Check sheet for the drawn part. Datum: minimum x, y, z corner. Units: mm. A direction names the side the tool comes from. Coordinates: 2 decimals unless noted, no trailing zeros. Loops run counter-clockwise (first coordinate to the right, second up) from the corner with the lowest first, then second, coordinate; pieces in that order, holes last.
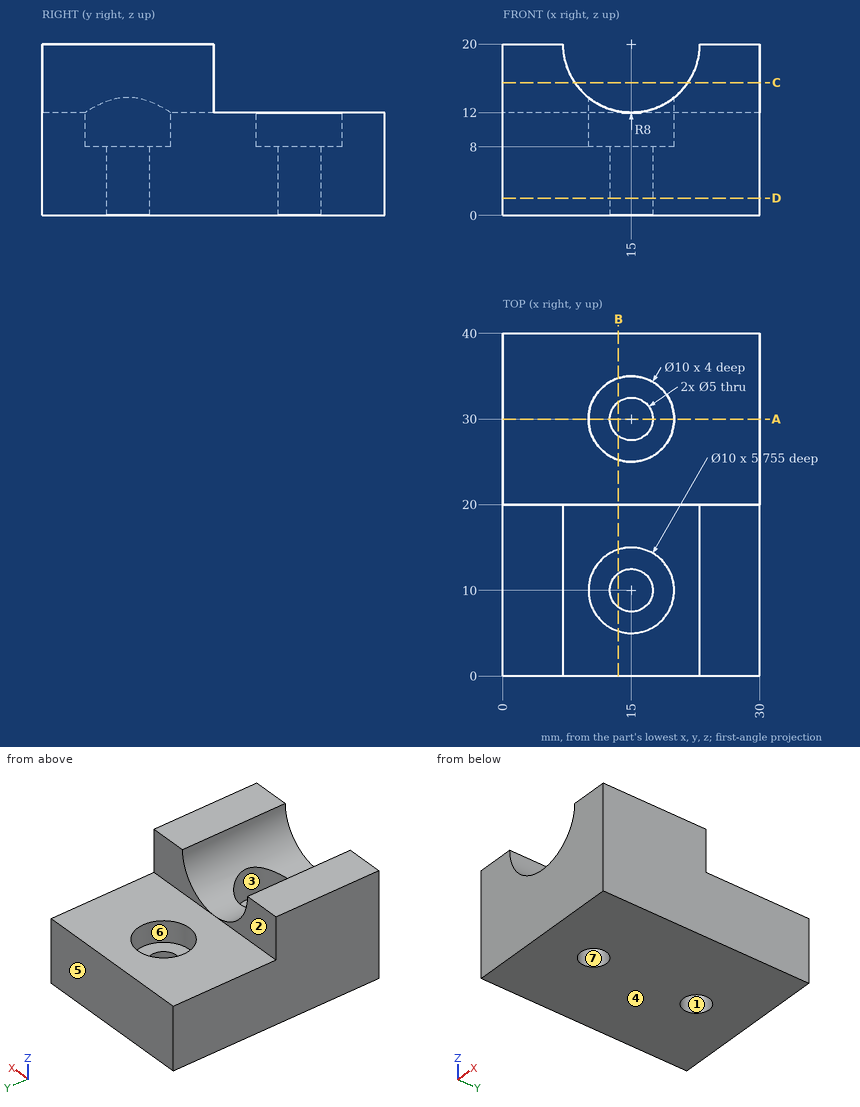
1) Mould release check, pull along Y, two halves, no side actions. Record for the marked faces 4, 5, 6 and 7: +Y half, -Y half, draft (parallel to the pull), parting line (faces both ways), or undercut.
Answer sheet:
face 4: draft
face 5: +Y half
face 6: undercut
face 7: undercut
2) Section check A-A on y = 30. Enter the section's corners in (x, z).
Answer sheet:
outline: (0, 0) - (12.5, 0) - (12.5, 8) - (10, 8) - (10, 12) - (0, 12) - close; (17.5, 0) - (30, 0) - (30, 12) - (20, 12) - (20, 8) - (17.5, 8) - close
3) Set-up check for the marked faces 1, 2 and 3: record each of +Z, -Z, +X, -X, +Y, -Y from which the full face is reachable in a straight line by a thin tool's end or side.
Answer sheet:
face 1: +Z, -Z
face 2: +Z, +X, -X, +Y
face 3: +Z
4) Scan lines: line 1 (Y direction, x = 15, z = 10.95); line 2 (Y direction, x = 15, z = 5.5); line 3 (Z direction, x = 24, y = 32). Record each from-to range of solid material in increasing order.
Answer sheet:
line 1: y = 0 to 5, 15 to 25, 35 to 40
line 2: y = 0 to 7.5, 12.5 to 27.5, 32.5 to 40
line 3: z = 0 to 12
5) Section check C-C on z = 15.5. Enter the section's corners in (x, y).
Answer sheet:
outline: (0, 0) - (8.39, 0) - (8.39, 20) - (0, 20) - close; (21.61, 0) - (30, 0) - (30, 20) - (21.61, 20) - close
6) Section check B-B on x = 13.5. Enter the section's corners in (y, z).
Answer sheet:
outline: (0, 0) - (8, 0) - (8, 8) - (5.23, 8) - (5.23, 12.14) - (0, 12.14) - close; (12, 0) - (28, 0) - (28, 8) - (25.23, 8) - (25.23, 12) - (20, 12) - (20, 12.14) - (14.77, 12.14) - (14.77, 8) - (12, 8) - close; (32, 0) - (40, 0) - (40, 12) - (34.77, 12) - (34.77, 8) - (32, 8) - close
7) Depth check by flat-ended pin: pin 1 (4 mm diameter, centred on x = 14, y = 22.5, fed in from +Z); pin 2 (1 mm diameter, centred on x = 9.5, z = 13.5, fed in from +Y); pin 3 (8 mm diameter, centred on x = 15, y = 30, fed in from +Z). Enter the tip coordinate at first touch or a pass-through.
Answer sheet:
pin 1: stops at z = 12
pin 2: stops at y = 20
pin 3: stops at z = 8
8) Section check D-D on z = 2. Enter the section's corners in (x, y).
Answer sheet:
outline: (0, 0) - (30, 0) - (30, 40) - (0, 40) - close; hole circle Ø5 at (15, 10); hole circle Ø5 at (15, 30)
